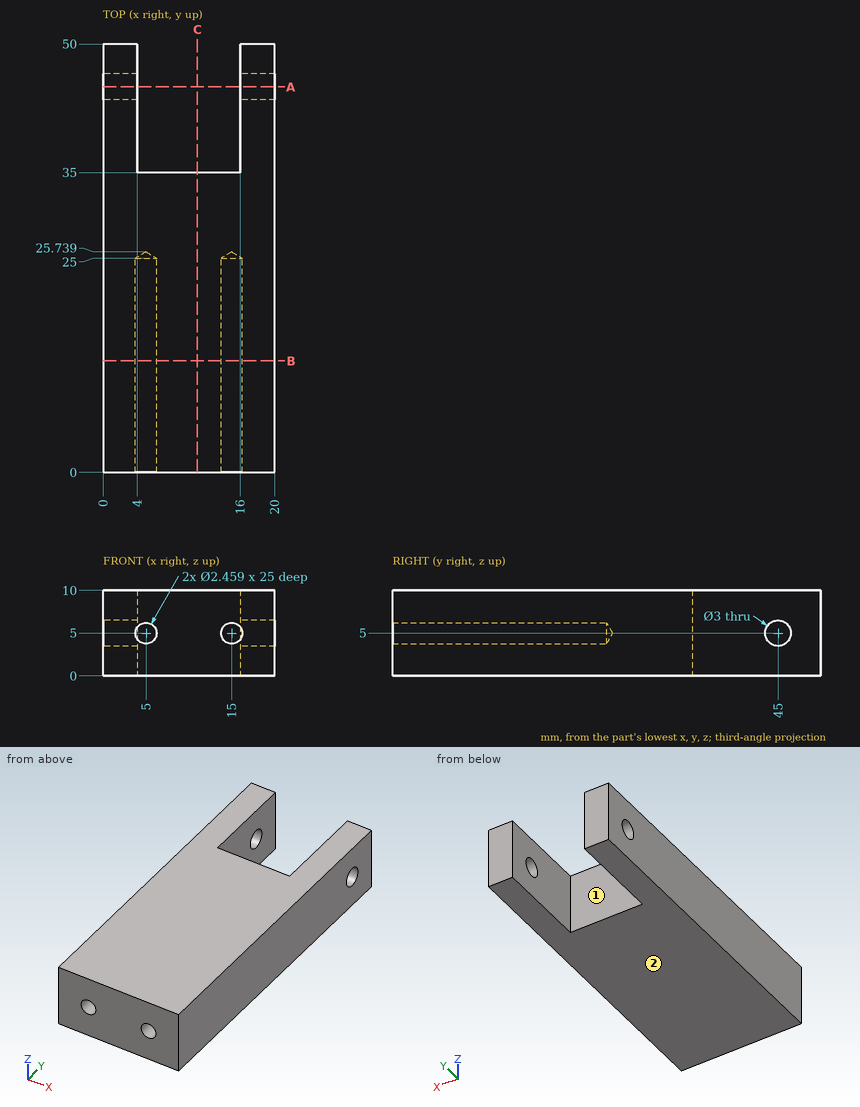
Check sheet for the drawn part. Datum: minimum x, y, z corner. Units: mm. A direction names the side the tool comes from. Coordinates: 2 decimals unless noted, no trailing zeros. Order: outer loops, then holes, each group sorted by start corner. A loop starts at its lowest first (then second) coordinate and runs counter-clockwise, first axis right, second up. Notation, with made-up numbers: M 8,25 L 48,25 A28 ccw 48,64 Z; hole C -5.75,-23 d3. An arc over 180 degrees is marked long. One line per question, with ' | ' between items. Start each with the question number.
Item 1: Access from +Z, -Z, +X, -X, +Y, -Y to the whole of each face (thin tool, end or side, straight path). Record for the marked faces 1 and 2.
Item 2: Sectioned sample at B-B on y = 13. Record the cut outline in (x, z), and give its area (4 significant figures).
Item 3: Material ranges on line 1 (X direction, y = 6.25, z = 5); line 2 (X direction, y = 47.5, z = 7.75); line 3 (Z direction, x = 2, y = 45), recorded low to high.
Item 4: Gauge pin test, flat ends, axial feed: P1, Ø2, axis at x = 8, z = 4, coming from the -Y side; P2, Ø5, axis at x = 9.5, z = 4.5, coming from the +Y side; P3, Ø2.5, axis at y = 45, z = 5, coming from the -X side. Record the tip position at first contact, or that the pin passes through.
Item 5: Sectioned sample at A-A on y = 45. Record the cut outline in (x, z), and give its area (3 significant figures).
Item 6: Sectioned sample at C-C on x = 11. Record the cut outline in (y, z), and give its area (3 significant figures).
Answer below:
1) face 1: +Z, -Z, +Y | face 2: -Z, +X, -X, +Y, -Y
2) outline: M 0,0 L 20,0 L 20,10 L 0,10 Z; hole C 5,5 d2.46; hole C 15,5 d2.46 | area: 190.5 mm^2
3) line 1: x = 0 to 3.77, 6.23 to 13.77, 16.23 to 20 | line 2: x = 0 to 4, 16 to 20 | line 3: z = 0 to 3.5, 6.5 to 10
4) P1: stops at y = 0 | P2: stops at y = 35 | P3: passes through
5) outline: M 0,0 L 4,0 L 4,3.5 L 0,3.5 Z; M 0,6.5 L 4,6.5 L 4,10 L 0,10 Z; M 16,0 L 20,0 L 20,3.5 L 16,3.5 Z; M 16,6.5 L 20,6.5 L 20,10 L 16,10 Z | area: 56.0 mm^2
6) outline: M 0,0 L 35,0 L 35,10 L 0,10 Z | area: 350 mm^2
